Part model, mm, in its own coordinate system. Give positions to 0.01 mm unless a question says otherwise; leave off trailing zeros. Loops run counter-clockwise (first coordinate to the right, second up) from the corner with the lowest first, then second, coordinate; pieces in that order, holes last. Notation, with made-up numbers: M 32.25,12 L 47.25,12 A23 ccw 47.25,31 Z; hole C -34,30 d4. An arc over 180 degrees is marked long. Put each result on its own line as item: value. Start each with the question number.
```python
from build123d import *

# Parameters (mm, degrees)
SKETCH2_R               = 5
CUT_EXTRUDE1_DEPTH      = 1
SKETCH3_W               = 1
SKETCH3_H               = 1
CUT_EXTRUDE2_DEPTH      = 12
CUT_EXTRUDE2_DEPTH_BACK = 6.5
SKETCH4_R               = 0.225
BOSS_EXTRUDE1_DEPTH     = 4.5


with BuildPart() as part:
    # Sketch1 → Revolve1 (revolve)
    with BuildSketch(Plane.XY):
        with BuildLine():
            Line((0, 0), (5.5, 0))
            Line((5.5, 0), (4.582575695, 11))
            ThreePointArc((4.582575695, 11), (2.883140649, 13.524917218), (0, 14.5))
            Line((0, 14.5), (0, 0))
        make_face()
    revolve(axis=Axis((0, 0, 0), (0, 1, 0)))

    # Sketch2 → Cut-Extrude1 (cut)
    with BuildSketch(Plane.XZ):
        Circle(SKETCH2_R)
    extrude(amount=-CUT_EXTRUDE1_DEPTH, mode=Mode.SUBTRACT)

    # Sketch3 → Cut-Extrude2 (cut, two sides)
    with BuildSketch(Plane.XY) as cut_extrude2_sk:
        Rectangle(SKETCH3_W, SKETCH3_H)
    extrude(amount=CUT_EXTRUDE2_DEPTH, mode=Mode.SUBTRACT)
    extrude(cut_extrude2_sk.sketch, amount=-CUT_EXTRUDE2_DEPTH_BACK, mode=Mode.SUBTRACT)

    # Sketch4 → Boss-Extrude1 (add)
    with BuildSketch(Plane.XZ.offset(-1)):
        with Locations((1.796051224, 1.796051224)):
            Circle(SKETCH4_R)
        with Locations((-1.796051224, 1.796051224)):
            Circle(SKETCH4_R)
        with Locations((-1.796051224, -1.796051224)):
            Circle(SKETCH4_R)
    extrude(amount=BOSS_EXTRUDE1_DEPTH)


solid = part.part
```
1) Band-saw the part on C-C on y = -1. Give the cut face in (x, z) (3 decimals).
2) Wall check: L1, parallel to X at y = 0.5, z = 0; L2, parallel to Z at x = 0, y = 0.55; L3, parallel to X at y = 0.8, z = 0. Give the ranges that are in metal, low to high.
3) Band-saw the part on D-D on y = 12. Give the cut face in (x, z), then the cut area to 3 significant figures.
4) Mould opens along X. For faces 1 (the flat face through (0, 1, 0)), 2 (the flat face through (-5.2, 0, 0)), 3 (the conical face through (4.802, 5.577, -1.512)) say: +X half, -X half, draft (parallel to the pull), parting line (faces both ways), or undercut.
5) Pin check, flat tips, straight feed: pin 1 Ø0.6 at (y, z) = (0, 5) entering from +X; pin 2 Ø1.5 at (x, y) = (-4, 1) entering from +Z; pin 3 Ø5 at (x, z) = (-2.5, 1.5) entering from -Y; pin 4 Ø6 at (y, z) = (11, -4) entering from +X. Stop position of each tip, or through.
6) Band-saw the part on A-A on z = 0. Give the cut face in (x, y), then the cut area to 3 significant figures.
7) Band-saw the part on B-B on x = 0. Give the cut face in (y, z).
Evaluation:
1. outline: C -1.796,-1.796 d0.45; C -1.796,1.796 d0.45; C 1.796,1.796 d0.45
2. L1: -5.46 to -5, 5 to 5.46
2. L2: -5.45 to -5, 5 to 5.45
2. L3: -5.43 to -5, 5 to 5.43
3. outline: C 0,0 d8.37
3. area: 55.0 mm2
4. face 1: undercut
4. face 2: draft
4. face 3: parting line
5. pin 1: x = 2.86
5. pin 2: z = 4.34
5. pin 3: y = -3.5
5. pin 4: x = 4.52
6. outline: M -5.5,0 L -5,0 L -5,1 L 5,1 L 5,0 L 5.5,0 L 4.58,11 A4.75 ccw -4.58,11 Z
6. area: 125 mm2
7. outline: M 0.5,-5.46 L 11,-4.58 A4.75 ccw 11,4.58 L 0.5,5.46 L 0.5,5 L 1,5 L 1,-5 L 0.5,-5 Z
